For this review, take the finished solid that the model builds, in its own axes (mm). Face numbers are marked on the shaded views. Coordinates: 2 decimals unless noted, no trailing zeros. Loops run counter-clockwise (first coordinate to the right, second up) from the corner with the lowest first, then second, coordinate; pieces in that order, holes last. Notation, with made-up numbers: M 5.25,38 L 43.25,38 A8 ccw 43.25,43 Z; hole C 51,5.25 d5. An arc over 180 degrees is marked long. Answer as a JSON object with one key per item and string values. Group by question number.
Item 1: Insertion check: pin 1 (2.5 mm diameter, centred on x = 0, y = 0, fed in from +Z). The pin has a flat end and moves straight along its axis. Give the tip position at first contact, or say it passes through.
Item 2: Wall thickness on L1, parallel to Y at x = 0, z = 2.45; L2, parallel to X at y = 1, z = 1.3; L3, parallel to Y at x = -0.5, z = 1.2: over which ranges is each line inside the solid? List them lowest first. Write a range as from..to.
Item 3: Add section C-C (z = 3.4). State the section outline as (x, y) points (3 decimals).
Item 4: Add section A-A (y = 0). State the section outline as (x, z) points.
Item 5: Add section B-B (z = 1.9). State the section outline as (x, y) points.
Item 6: Mouldability with a two-part tool opening along X and no side actions: class the marked faces 1, 2 and 3 as +X half, -X half, draft (parallel to the pull), parting line (faces both ways), or undercut.
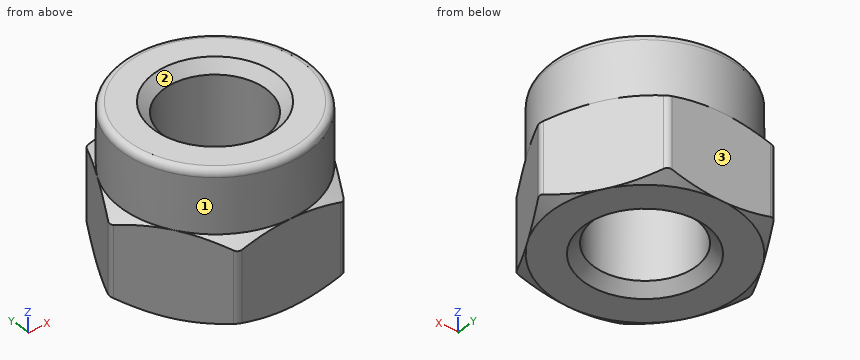
from build123d import *

# Parameters (mm, degrees)
EXTRUDE_307_DEPTH     = 2.5
SKETCH_2_R            = 2.75
EXTRUDE_489_DEPTH     = 1.8
SKETCH_3_R            = 1.5
CUT_EXTRUDE_587_DEPTH = 7.011308787
FILLET_2_R            = 0.2
CHAMFER_1_SIZE        = 0.3
CHAMFER_2_SIZE        = 0.3
FILLET_3_R            = 0.2


with BuildPart() as part:
    # 草图1 → Extrude 307 (new body)
    with BuildSketch(Plane.XY):
        Polygon((3.175426481, 0), (1.58771324, 2.75), (-1.58771324, 2.75), (-3.175426481, 0), (-1.58771324, -2.75), (1.58771324, -2.75), align=None)
    extrude(amount=EXTRUDE_307_DEPTH)

    # 草图2 → Extrude 489 (add)
    with BuildSketch(Plane.XY.offset(2.5)):
        with Locations(Location((0, 0, 0), (0, 0, 150))):
            Circle(SKETCH_2_R)
    extrude(amount=EXTRUDE_489_DEPTH)

    # 草图3 → Cut-Extrude 587 (cut, through all)
    with BuildSketch(Plane.XY.offset(4.3)):
        Circle(SKETCH_3_R)
    extrude(amount=-CUT_EXTRUDE_587_DEPTH, mode=Mode.SUBTRACT)

    # 圆角2
    fillet_2_edges = [part.edges().sort_by_distance(p)[0] for p in [
        (1.58771324, -2.75, 1.25),
        (-1.58771324, -2.75, 1.25),
        (-3.175426481, 0, 1.25),
        (-1.58771324, 2.75, 1.25),
        (1.58771324, 2.75, 1.25),
        (3.175426481, 0, 1.25),
    ]]
    fillet(fillet_2_edges, radius=FILLET_2_R)

    # 倒角1
    chamfer_1_edges = [part.edges().sort_by_distance(p)[0] for p in [
        (-1.5, 0, 0),
    ]]
    chamfer(chamfer_1_edges, length=CHAMFER_1_SIZE)

    # 倒角2
    chamfer_2_edges = [part.edges().sort_by_distance(p)[0] for p in [
        (-1.5, 0, 4.3),
    ]]
    chamfer(chamfer_2_edges, length=CHAMFER_2_SIZE)

    # 草图6 → 切除-旋转2 (revolve, cut)
    with BuildSketch(Plane(origin=(0, 0, 0), x_dir=(1, 0, 0), z_dir=(0, 1, 0))):
        Polygon((-2.75, 0), (-3.144486373, -0.227756814), (-3.144486373, 0), align=None)
        Polygon((-3.144486373, -2.5), (-3.144486373, -2.272243186), (-2.75, -2.5), align=None)
    revolve(axis=Axis((0, 0, -1.923239397), (0, 0, 1)), mode=Mode.SUBTRACT)

    # 圆角3
    fillet_3_edges = [part.edges().sort_by_distance(p)[0] for p in [
        (2.38156986, -1.375, 4.3),
    ]]
    fillet(fillet_3_edges, radius=FILLET_3_R)


solid = part.part
From the geometry:
{
 "1": {"pin 1": "passes through"},
 "2": {"L1": "y = -2.75..-1.5, 1.5..2.75", "L2": "x = -2.6..-1.12, 1.12..2.6", "L3": "y = -2.75..-1.41, 1.41..2.75"},
 "3": {"outline": "C 0,0 d5.5; hole C 0,0 d3"},
 "4": {"outline": "M -3.14,0.23 L -2.75,0 L -1.8,0 L -1.5,0.3 L -1.5,4 L -1.8,4.3 L -2.55,4.3 A0.2 ccw -2.75,4.1 L -2.75,2.5 L -3.14,2.27 Z; M 1.5,0.3 L 1.8,0 L 2.75,0 L 3.14,0.23 L 3.14,2.27 L 2.75,2.5 L 2.75,4.1 A0.2 ccw 2.55,4.3 L 1.8,4.3 L 1.5,4 Z"},
 "5": {"outline": "M -3.12,-0.1 L -1.65,-2.65 A0.2 ccw -1.47,-2.75 L 1.47,-2.75 A0.2 ccw 1.65,-2.65 L 3.12,-0.1 A0.2 ccw 3.12,0.1 L 1.65,2.65 A0.2 ccw 1.47,2.75 L -1.47,2.75 A0.2 ccw -1.65,2.65 L -3.12,0.1 A0.2 ccw Z; hole C 0,0 d3"},
 "6": {"face 1": "parting line", "face 2": "undercut", "face 3": "draft"}
}
